```python
from build123d import *

# Parameters (mm, degrees)
EXTRUDE_1_DEPTH         = 200
HOLE_WIZARD_6_0_6_6_D   = 6
HOLE_WIZARD_5_5_5_5_1_D = 5.5


with BuildPart() as part:
    # Sketch1 → 凸台-拉伸1 (new body)
    with BuildSketch(Plane.XY):
        Polygon((-6.5, 45), (-3.2, 45), (-3.2, 43.2), (-5.1, 43.2), (-5.1, 37.2), (5.1, 37.2), (5.1, 43.2), (3.2, 43.2), (3.2, 45), (6.5, 45), (7.5, 45), (7.5, 44), (7.5, 18.2), (5, 18.2), (5, 20.2), (-0.5, 20.2), (-0.5, 18.2), (-3, 18.2), (-3, 11.8), (-0.5, 11.8), (-0.5, 9.8), (5, 9.8), (5, 11.8), (7.5, 11.8), (7.5, -11.8), (5, -11.8), (5, -9.8), (-0.5, -9.8), (-0.5, -11.8), (-3, -11.8), (-3, -18.2), (-0.5, -18.2), (-0.5, -20.2), (5, -20.2), (5, -18.2), (7.5, -18.2), (7.5, -44), (7.5, -45), (6.5, -45), (3.2, -45), (3.2, -43.2), (5.1, -43.2), (5.1, -37.2), (-5.1, -37.2), (-5.1, -43.2), (-3.2, -43.2), (-3.2, -45), (-6.496721962, -45), (-7.5, -45), (-7.5, -44), (-7.5, -33.2), (-5, -33.2), (-5, -35.2), (0.5, -35.2), (0.5, -33.2), (3, -33.2), (3, -26.8), (0.5, -26.8), (0.5, -24.8), (-5, -24.8), (-5, -26.8), (-7.5, -26.8), (-7.5, -3.2), (-5, -3.2), (-5, -5.2), (0.5, -5.2), (0.5, -3.2), (3, -3.2), (3, 3.2), (0.5, 3.2), (0.5, 5.2), (-5, 5.2), (-5, 3.2), (-7.5, 3.2), (-7.5, 26.8), (-5, 26.8), (-5, 24.8), (0.5, 24.8), (0.5, 26.8), (3, 26.8), (3, 33.2), (0.5, 33.2), (0.5, 35.2), (-5, 35.2), (-5, 33.2), (-7.5, 33.2), (-7.5, 44), (-7.5, 45), align=None)
    extrude(amount=EXTRUDE_1_DEPTH)

    # Ø6.0 (6) 直径孔6 (through all)
    with Locations(Plane(origin=(7.5, 0, 0), x_dir=(0, 0, -1), z_dir=(1, 0, 0))):
        with Locations((-158, -30), (-158, 30), (-122, -30), (-122, 30), (-54, 30), (-54, -30), (-18, -30), (-18, 30), (-106, 0), (-70, 0)):
            Hole(HOLE_WIZARD_6_0_6_6_D / 2)

    # Ø5.5 (5.5) 直径孔1 (through all)
    with Locations(Plane(origin=(-3, 0, 0), x_dir=(0, 0, -1), z_dir=(1, 0, 0))):
        with Locations((-193, -15), (-193, 15), (-7, -15), (-7, 15)):
            Hole(HOLE_WIZARD_5_5_5_5_1_D / 2)


solid = part.part
```
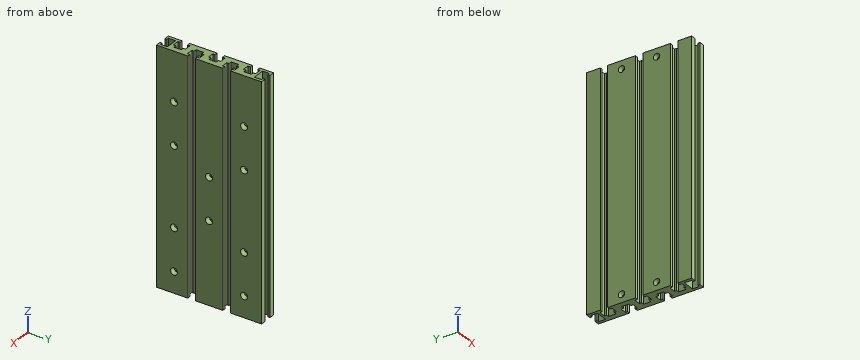
Can you work these out from the model? Positions are in its coordinate system, mm. Give positions to 0.01 mm unless a question says otherwise; leave off trailing zeros. Loops run counter-clockwise (first coordinate to the right, second up) from the corner with the lowest first, then second, coordinate; pieces in that order, holes last. Notation, with made-up numbers: M 85,68.5 L 139,68.5 A28 ccw 139,90.5 Z; hole C 23,53 d10. An arc over 180 degrees is marked long. Use one line per item in the form item = value. Start each with the question number.
(1) I want a section at C-C, the plane y = -15. Write out the boundary of the cut face in (x, z), and give its area (4 significant figures).
(2) I'm going to push flat-ended pins straight in: P1, Ø2, axis at x = 2, z = 66.5, coming from the +Y side; P2, Ø5, axis at x = 0, z = 87, coming from the -Y side; P3, Ø3, axis at y = -15, z = 149.5, coming from the +X side; P4, Ø4, axis at y = -31.5, z = 140.5, coming from the -X side. Where does each tip first touch, or does it pass through?
(3) I want a section at A-A, the plane y = 0. Write out the boundary of the cut face in (x, z).
(4) I want a section at B-B, the plane z = 54. State how many separate pieces and enclosed holes the cut face has, and give its area (3 significant figures).
(5) Please list where these lines run through material, in increasing order: line 1 (Y direction, x = -1.75, z = 174.5); line 2 (Y direction, x = 4.5, z = 8.5); line 3 (Y direction, x = 5.5, z = 44.5).
Worked out:
q1.outline = M -7.5,0 L -3,0 L -3,4.25 L -7.5,4.25 Z; M -7.5,9.75 L -3,9.75 L -3,190.25 L -7.5,190.25 Z; M -7.5,195.75 L -3,195.75 L -3,200 L -7.5,200 Z
q1.area = 850.5 mm²
q2.P1 = 37.2
q2.P2 = -37.2
q2.P3 = -3
q2.P4 = -7.5
q3.outline = M 3,0 L 7.5,0 L 7.5,67 L 3,67 Z; M 3,73 L 7.5,73 L 7.5,103 L 3,103 Z; M 3,109 L 7.5,109 L 7.5,200 L 3,200 Z
q4.separate_pieces = 3
q4.enclosed_holes = 0
q4.area = 705 mm²
q5.line_1 = -37.2 to -35.2, -24.8 to -18.2, -11.8 to -5.2, 5.2 to 11.8, 18.2 to 24.8, 35.2 to 37.2
q5.line_2 = -45 to -43.2, -37.2 to -20.2, -9.8 to 9.8, 20.2 to 37.2, 43.2 to 45
q5.line_3 = -45 to -18.2, -11.8 to 11.8, 18.2 to 45
